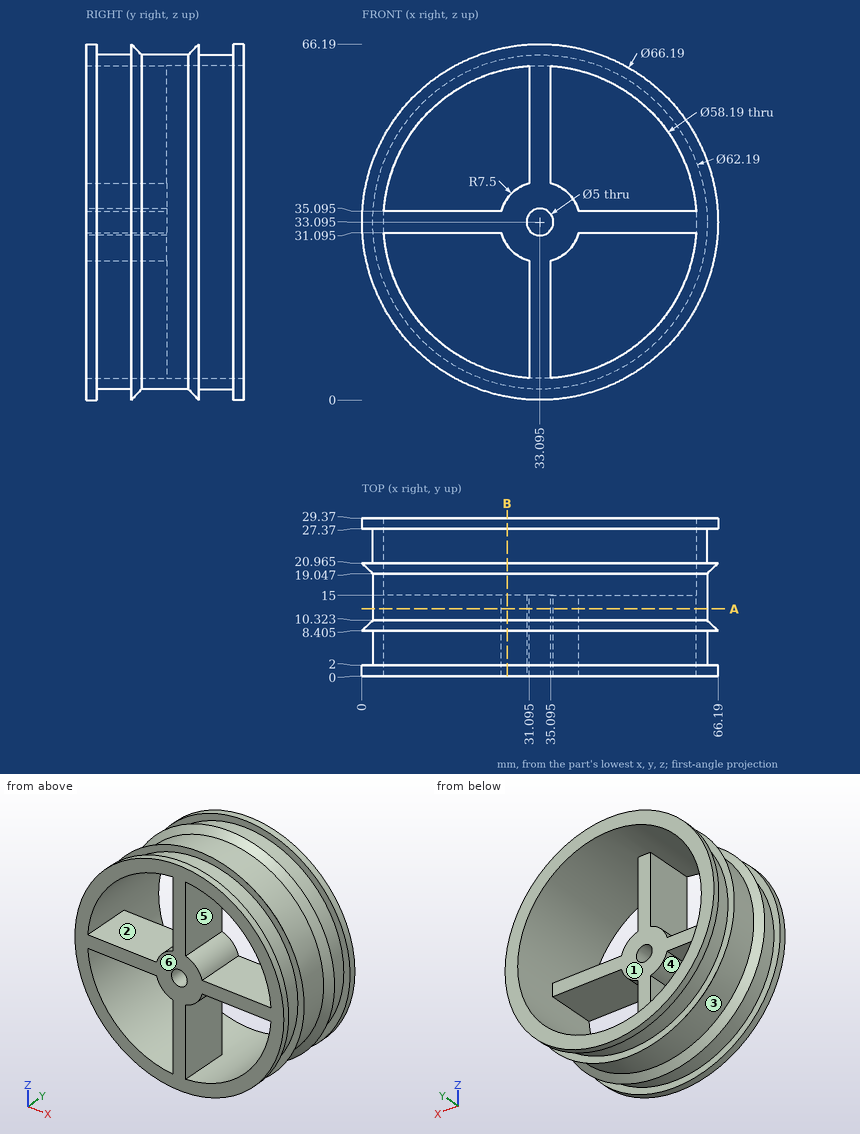
Answer from the drawing. Dimensions are ordinates in mm from the lowest x, y and z of the part. A direction names the side the tool comes from. Give positions to 0.01 mm unless a question says otherwise; leave off trailing zeros. Order: outer loops, then holes, each group sorted by start corner. A loop starts at its lowest first (then second) coordinate and runs counter-clockwise, first axis right, second up.
Item 1: Given pin 1 Ø16.5 at (x, y) = (10, 5.5) entering from -Z; pin 2 Ø1.5 at (y, z) = (7, 40) entering from -X (1 decimal); pin 3 Ø1.5 at (x, y) = (10, 10) entering from -Z, each flat-ended and moving along its own axis, determine where each tip first touches the part or whether it passes through.
From the geometry:
pin 1: stops at z = 3.79
pin 2: stops at x = 2.6
pin 3: stops at z = 10.4
Item 2: Find the intervals of material crossed by probe 1 along Z at (x, y) = (38.5, 9) (1 decimal); probe 2 along Y at (x, z) = (7, 52) (1 decimal); probe 3 along Y at (x, z) = (57, 12) (1 decimal), in increasing order.
From the geometry:
probe 1: z = 1.1 to 4.5, 27.9 to 38.3, 61.7 to 65.1
probe 2: y = 0 to 2, 8.4 to 9.2, 20.1 to 21, 27.4 to 29.4
probe 3: y = 0 to 2, 8.4 to 9.6, 19.8 to 21, 27.4 to 29.4
Item 3: The part is cut by section A-A, the plane y = 12.5. Give the vertices of the cut face in (x, z) (1 decimal).
From the geometry:
outline: circle Ø62.2 at (33.1, 33.1); hole (4.1, 31.1) arc R29.1 ccw to (31.1, 4.1) - (31.1, 25.9) arc R7.5 cw to (25.9, 31.1) - close; hole (4.1, 35.1) - (25.9, 35.1) arc R7.5 cw to (31.1, 40.3) - (31.1, 62.1) arc R29.1 ccw to start; hole circle Ø5 at (33.1, 33.1); hole (35.1, 4.1) arc R29.1 ccw to (62.1, 31.1) - (40.3, 31.1) arc R7.5 cw to (35.1, 25.9) - close; hole (35.1, 40.3) arc R7.5 cw to (40.3, 35.1) - (62.1, 35.1) arc R29.1 ccw to (35.1, 62.1) - close
Item 4: For a pull along X with two mould halves and no side action, classify the marked faces 3, 4, 5 and 6 as pulls with the +X half, pulls with the -X half, needs draft (parallel to the pull), parting line crosses it, or undercut.
From the geometry:
face 3: parting line crosses it
face 4: undercut
face 5: undercut
face 6: needs draft
Item 5: Which of the six approach directions +Z, -Z, +X, -X, +Y, -Y give full straight-line access (tool end or side, diameter ignored) to the marked faces 1 and 2?
From the geometry:
face 1: +Y
face 2: +Y, -Y
Item 6: The part is cut by section B-B, the plane x = 27. Count the separate pieces of the cut face and the enclosed holes in it, and give its area (3 significant figures).
From the geometry:
separate pieces: 3
enclosed holes: 0
area: 275 mm2
